from build123d import *

# Parameters (mm, degrees)
F0_W      = 68
F0_H      = 64.6
F1_DEPTH  = 20
F2_R      = 2
F3_W      = 3
F3_H      = 6.8213130001
F4_DEPTH  = 2
F5_W      = 3
F5_H      = 2.5574813623
F6_DEPTH  = 5
F7_R      = 0.5
F8_DEPTH  = 25
F9_W      = 64
F9_H      = 60.6
F9_R      = 2.5
F10_DEPTH = 1


with BuildPart() as f1:
    # F0 (on Top) → F1 (new body)
    with BuildSketch(Plane.XY):
        with Locations((34, -32.3)):
            Rectangle(F0_W, F0_H)
    extrude(amount=F1_DEPTH)

    # F2
    f2_edges = [f1.edges().sort_by_distance(p)[0] for p in [
        (34, 0, 20),
        (0, -32.3, 20),
        (34, -64.6, 20),
        (68, -32.3, 20),
        (34, 0, 0),
        (0, -32.3, 0),
        (34, -64.6, 0),
        (68, -32.3, 0),
        (68, -64.6, 10),
        (68, 0, 10),
        (0, 0, 10),
        (0, -64.6, 10),
    ]]
    fillet(f2_edges, radius=F2_R)

    # F3 (on face) → F4 (cut)
    with BuildSketch(Plane.XY.offset(20)):
        with Locations((5.5, -11.5893434999)):
            Rectangle(F3_W, F3_H)
    extrude(amount=-F4_DEPTH, mode=Mode.SUBTRACT)

    # F5 (on face) → F6 (join)
    with BuildSketch(Plane.XY.offset(18)):
        with Locations((5.5, -9.457427681)):
            Rectangle(F5_W, F5_H)
    extrude(amount=F6_DEPTH)

    # F7 (on face) → F8 (join)
    with BuildSketch(Plane(origin=(0, 0, 0), x_dir=(0, -1, 0), z_dir=(-1, 0, 0))):
        with Locations((54.3, 14.6)):
            Circle(F7_R)
        with Locations((55.4, 14.6)):
            Circle(F7_R)
    extrude(amount=F8_DEPTH)

    # F9 (on face) → F10 (cut)
    with BuildSketch(Plane(origin=(0, 0, 0), x_dir=(1, 0, 0), z_dir=(0, 0, -1))):
        with Locations((34, 32.3)):
            Rectangle(F9_W, F9_H)
        with Locations((6, 32.3)):
            Circle(F9_R, mode=Mode.SUBTRACT)
        with Locations((6, 32.3)):
            Circle(F9_R)
    extrude(amount=-F10_DEPTH, mode=Mode.SUBTRACT)


solid = f1.part
CAD build for the part. Positions are in the model's coordinates, mm. A direction names the side the tool comes from. Give positions to 0.01 mm unless a question says otherwise; leave off trailing zeros. Loops run counter-clockwise (first coordinate to the right, second up) from the corner with the lowest first, then second, coordinate; pieces in that order, holes last. Notation, with made-up numbers: M 11,-10 L 38,-10 A23 ccw 38,5 Z; hole C 66,-19.75 d9. An arc over 180 degrees is marked long. Answer in a Markdown table with one row per item. Add a question column.
Item 1: Probe probe 1 along Z at (x, y) = (60.5, -6.5); probe 2 along X at (y, z) = (-29, 14.25); probe 3 along Z at (x, y) = (5, -14). List the from-to ranges inside material, lowest first.
Item 2: Drop flat-ended pins along their axis: P1, Ø1.5, axis at y = -22, z = 12.5, coming from the -X side; P2, Ø1.5, axis at x = 6, z = 21.5, coming from the +Y side; P3, Ø18, axis at x = 43.5, y = -33.5, coming from the +Z side; P4, Ø5, axis at x = 4, y = -51.5, coming from the -Z side. Give the stop position or say it passes through.
Item 3: Band-saw the part on D-D on x = -2.5. Give the cut face in (y, z), then the cut area to 3 significant figures.
Item 4: Band-saw the part on B-B on x = 55.5. Give the cut face in (y, z).
Item 5: Tool access for faces 1 (the face through (5, -8.179, 21)), 2 (the face through (7, -13, 19)), 3 (the face through (5, -9, 23)), 4 (the face through (4, -9, 21)): list every direction of +Z, -Z, +X, -X, +Y, -Y with a clear straight run to the whole face (end or side of a thin tool).
Item 6: Mould opens along X. For faces 5 (the face through (5, -13, 18)), 6 (the face through (34.45, -64.03, 0.6)), 7 (the face through (67.43, -31.88, 19.4)), 8 (the face through (34, -33, 1)) say: +X half, -X half, draft (parallel to the pull), parting line (faces both ways), or undercut.
Item 7: Band-saw the part on C-C on z = 3.75. Give the cut face in (x, y), then the cut area to 3 significant figures.
Item 8: Band-saw the part on A-A on y = -17. Give the cut face in (x, z).
Reply:
| question | item | result |
|---|---|---|
| 1 | probe 1 | z = 1 to 20 |
| 1 | probe 2 | x = 0 to 68 |
| 1 | probe 3 | z = 1 to 18 |
| 2 | P1 | stops at x = 0 |
| 2 | P2 | stops at y = -8.18 |
| 2 | P3 | stops at z = 20 |
| 2 | P4 | stops at z = 0 |
| 3 | outline | C -55.4,14.6 d1; C -54.3,14.6 d1 |
| 3 | area | 1.57 mm^2 |
| 4 | outline | M -64.6,2 A2 ccw -62.6,0 L -62.6,1 L -2,1 L -2,0 A2 ccw 0,2 L 0,18 A2 ccw -2,20 L -62.6,20 A2 ccw -64.6,18 Z |
| 5 | face 1 | +Z, +X, -X, +Y |
| 5 | face 2 | +Z |
| 5 | face 3 | +Z, +X, -X, +Y, -Y |
| 5 | face 4 | +Z, -X, +Y, -Y |
| 6 | face 5 | undercut |
| 6 | face 6 | draft |
| 6 | face 7 | +X half |
| 6 | face 8 | undercut |
| 7 | outline | M 0,-62.6 A2 ccw 2,-64.6 L 66,-64.6 A2 ccw 68,-62.6 L 68,-2 A2 ccw 66,0 L 2,0 A2 ccw 0,-2 Z |
| 7 | area | 4,390 mm^2 |
| 8 | outline | M 0,2 A2 ccw 2,0 L 2,1 L 66,1 L 66,0 A2 ccw 68,2 L 68,18 A2 ccw 66,20 L 2,20 A2 ccw 0,18 Z |
